Geometry: final body of the model. Coordinates: model frame, mm. Face numbers are marked on the shaded views. A direction names the side the tool comes from. Give positions to 0.01 mm unless a question says otherwise; leave off trailing zeros. Write each loop counter-clockwise with the first axis right and the second up, starting at its lowest first coordinate (ties: lowest second). Pieces come first, ordered by that corner, then holes. Notation, with made-up numbers: M 49,-35 L 81,-35 A13 cw 81,-17 Z; hole C 28.25,-6.5 d6. An arc over 180 degrees is marked long. Answer as a JSON object with one key per item and string values.
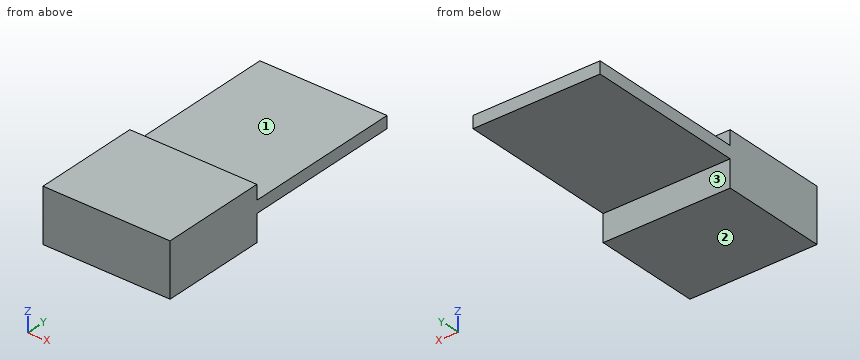
from build123d import *

# Parameters (mm, degrees)
F0_W     = 26.19
F0_H     = 33
F1_DEPTH = 2.5
F0_H_2   = 22
F2_DEPTH = 5.5
F3_DEPTH = 5.5


with BuildPart() as f1:
    # F0 (on Top) → F1 (new body)
    with BuildSketch(Plane.XY):
        with Locations((0, 11)):
            Rectangle(F0_W, F0_H)
    extrude(amount=F1_DEPTH)

    # F0 (on Top) → F2 (join)
    with BuildSketch(Plane.XY):
        with Locations((0, -16.5)):
            Rectangle(F0_W, F0_H_2)
    extrude(amount=F2_DEPTH)

    # F0 (on Top) → F3 (join)
    with BuildSketch(Plane.XY):
        with Locations((0, -16.5)):
            Rectangle(F0_W, F0_H_2)
    extrude(amount=-F3_DEPTH)


solid = f1.part
1) Cut plane C-C on y = 9. Return loops of the section in (x, z) (3 decimals).
Geometry check:
{"outline": "M -13.095,0 L 13.095,0 L 13.095,2.5 L -13.095,2.5 Z"}
2) Line query: line 1 (Z direction, x = 1, y = 0); line 2 (Y direction, x = 6, z = 4). Output: solid intervals per line, ascending. Write a range as from..to.
Geometry check:
{"line 1": "z = 0..2.5", "line 2": "y = -27.5..-5.5"}
3) Set-up query: the marked faces 1, 2 and 3. Return all of +Z, -Z, +X, -X, +Y, -Y with unobstructed straight access to the full face (end or side cutting, diameter ignored); none if empty.
Geometry check:
{"face 1": "+Z, +X, -X, +Y", "face 2": "-Z, +X, -X, +Y, -Y", "face 3": "-Z, +X, -X, +Y"}
4) Cut plane A-A on x = -7. Return loops of the section in (y, z), and give its area (4 significant figures).
Geometry check:
{"outline": "M -27.5,-5.5 L -5.5,-5.5 L -5.5,0 L 27.5,0 L 27.5,2.5 L -5.5,2.5 L -5.5,5.5 L -27.5,5.5 Z", "area": "324.5 mm2"}
5) Contact query for flat-ended pins moving along their axis: P1, Ø3, axis at x = 0, z = -3, coming from the +Y side; P2, Ø8, axis at x = 3, y = 8, coming from the -Z side; P3, Ø1.5, axis at x = -3.5, y = 11.5, coming from the +Z side. Output: stop coordinate, or through.
Geometry check:
{"P1": "stops at y = -5.5", "P2": "stops at z = 0", "P3": "stops at z = 2.5"}
6) Cut plane B-B on z = -3.5. Return loops of the section in (x, y) (3 decimals), and give its area (3 significant figures).
Geometry check:
{"outline": "M -13.095,-27.5 L 13.095,-27.5 L 13.095,-5.5 L -13.095,-5.5 Z", "area": "576 mm2"}
